Source: CAD feature listing. Evaluate the final solid. Frame: model axes, mm. Give positions to 0.01 mm unless a question says otherwise; leave off trailing zeros. Write each loop counter-clockwise with the first axis right and the second up, starting at its lowest first coordinate (ties: lowest second). Pieces come first, ordered by that corner, then holes.
```python
from build123d import *

# Parameters (mm, degrees)
SKETCH_1_W      = 800
SKETCH_1_H      = 1000
EXTRUDE_1_DEPTH = 20
SHELL_1_T       = -1.8


with BuildPart() as part:
    # 草图1 → 凸台-拉伸1 (new body)
    with BuildSketch(Plane.XY):
        with Locations((400, 500)):
            Rectangle(SKETCH_1_W, SKETCH_1_H)
    extrude(amount=EXTRUDE_1_DEPTH)

    # 抽壳1
    shell_1_openings = [part.faces().sort_by_distance(p)[0] for p in [
        (400, 500, 0),
    ]]
    offset(amount=SHELL_1_T, openings=shell_1_openings, kind=Kind.INTERSECTION)


solid = part.part
```
1. Pull-direction query (X, two-part tool) for faces 1 (the flat face through (0, 493, 10)), 2 (the flat face through (394, 507, 20)), 3 (the flat face through (800, 493, 10)), 4 (the flat face through (394, 507, 18.2)); classes: pulls with the +X half, pulls with the -X half, needs draft (parallel to the pull), parting line crosses it, or undercut.
2. Section query A-A (z = 5.5). Return loops of the section in (x, y), plus the area to 3 significant figures.
3. Line query: probe 1 along X at (y, z) = (688, 16); probe 2 along Y at (x, z) = (61.5, 3.5); probe 3 along Z at (x, y) = (576, 607). Output: solid intervals per line, ascending.
4. Pin query (flat end, axial travel): P1, Ø12, axis at x = 437, y = 161, coming from the -Z side. Return the tip coordinate at first contact, or that it passes through.
5. Section query B-B (x = 685). Return loops of the section in (y, z), plus the area to 3 significant figures.
6. Section query C-C (y = 134.5). Return loops of the section in (x, z).
The answers:
1. face 1: pulls with the -X half
1. face 2: needs draft
1. face 3: pulls with the +X half
1. face 4: undercut
2. outline: (0, 0) - (800, 0) - (800, 1000) - (0, 1000) - close; hole (1.8, 1.8) - (798.2, 1.8) - (798.2, 998.2) - (1.8, 998.2) - close
2. area: 6,470 mm2
3. probe 1: x = 0 to 1.8, 798.2 to 800
3. probe 2: y = 0 to 1.8, 998.2 to 1000
3. probe 3: z = 18.2 to 20
4. P1: stops at z = 18.2
5. outline: (0, 0) - (1.8, 0) - (1.8, 18.2) - (998.2, 18.2) - (998.2, 0) - (1000, 0) - (1000, 20) - (0, 20) - close
5. area: 1,870 mm2
6. outline: (0, 0) - (1.8, 0) - (1.8, 18.2) - (798.2, 18.2) - (798.2, 0) - (800, 0) - (800, 20) - (0, 20) - close
